Can you work these out from the model? Positions are in its coordinate system, mm. Face numbers are marked on the shaded views. A direction names the side the tool comes from. Give positions to 0.01 mm unless a question says otherwise; leave off trailing zeros. Order: outer loops, then holes, each group sorted by start corner. A loop starts at its lowest first (then second) coordinate and runs counter-clockwise, first axis right, second up.
Item 1: I want a section at B-B, the plane z = 13.25. Write out the boundary of the cut face in (x, y).
Item 2: I want a section at A-A, the plane x = 19. Write out the boundary of the cut face in (y, z).
Item 3: I'm going to push flat-ended pins straight in: pin 1 Ø1 at (x, y) = (-26.5, -22.5) entering from +Z; pin 2 Ø4 at (x, z) = (-13.5, 4) entering from -Y; pin 3 Ø4 at (y, z) = (-19.5, 7.5) entering from -X; pin 4 Ø1.1 at (x, y) = (43.5, 20.5) entering from -Z. Where does each tip first touch, or does it pass through?
Item 4: If I drill on line 1 along Y through (x, z) = (19, 0.7); line 2 along Y through (x, z) = (31, 10.75); line 3 along Z through (x, y) = (-11.5, -1), over which ranges is the centre line in solid material (lowest first)?
Item 5: If we mould it in two halves opening along Y, with no side actions, what happens to the marked faces 1, 2 and 3? For each: +Y half, -Y half, draft (parallel to the pull), parting line (faces both ways), or undercut.
Item 6: I want a section at D-D, the plane x = 38. Write out the boundary of the cut face in (y, z).
Item 7: I want a section at C-C, the plane y = -4. Write out the boundary of the cut face in (x, z), then the cut area to 3 significant figures.
Item 8: Which directions (+Z, -Z, +X, -X, +Y, -Y) give clear straight access to the entire face, cutting with the end or side of a thin tool? Please do the marked faces 4, 5, 6 and 7.
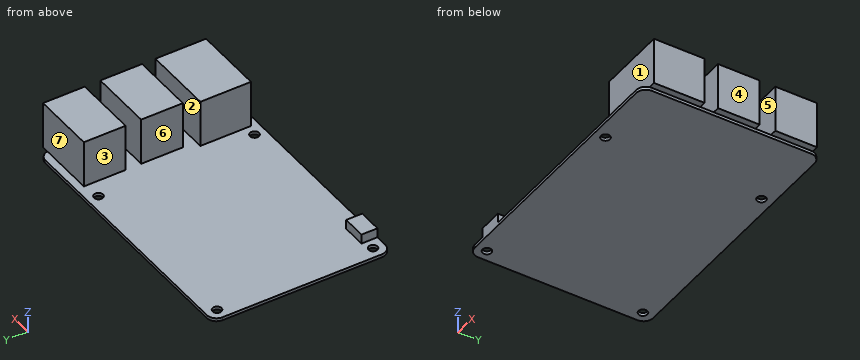
```python
from build123d import *

# Parameters (mm, degrees)
F0_W     = 85
F0_H     = 56
F1_DEPTH = 1
F2_R     = 3
F3_W     = 22
F3_H     = 15.9
F3_W_2   = 20
F3_H_2   = 13.1
F4_DEPTH = 14.8
F6_D     = 2.8
F6_DEPTH = 5
F7_W     = 7.5
F7_H     = 5
F8_DEPTH = 3


with BuildPart() as f1:
    # F0 (on Top) → F1 (new body)
    with BuildSketch(Plane.XY):
        Rectangle(F0_W, F0_H)
    extrude(amount=F1_DEPTH)

    # F2
    f2_edges = [f1.edges().sort_by_distance(p)[0] for p in [
        (42.5, -28, 0.5),
        (42.5, 28, 0.5),
        (-42.5, 28, 0.5),
        (-42.5, -28, 0.5),
    ]]
    fillet(f2_edges, radius=F2_R)

    # F3 (on face) → F4 (join)
    with BuildSketch(Plane.XY.offset(1)):
        with Locations((33.6, -17.75)):
            Rectangle(F3_W, F3_H)
        with Locations((34.6, 0.95)):
            Rectangle(F3_W_2, F3_H_2)
        with Locations((34.6, 18.95)):
            Rectangle(F3_W_2, F3_H_2)
    extrude(amount=F4_DEPTH)

    # F6
    with Locations(Plane.XY.offset(1)):
        with Locations((-39, 24.5), (19, 24.5), (19, -24.5), (-39, -24.5)):
            Hole(F6_D / 2, depth=F6_DEPTH)

    # F7 (on face) → F8 (join)
    with BuildSketch(Plane.XY.offset(1)):
        with Locations((-31.95, -25.5)):
            Rectangle(F7_W, F7_H)
    extrude(amount=F8_DEPTH)


solid = f1.part
```
Results list:
1. outline: (22.6, -25.7) - (44.6, -25.7) - (44.6, -9.8) - (22.6, -9.8) - close; (24.6, -5.6) - (44.6, -5.6) - (44.6, 7.5) - (24.6, 7.5) - close; (24.6, 12.4) - (44.6, 12.4) - (44.6, 25.5) - (24.6, 25.5) - close
2. outline: (-28, 0) - (-25.9, 0) - (-25.9, 1) - (-28, 1) - close; (-23.1, 0) - (23.1, 0) - (23.1, 1) - (-23.1, 1) - close; (25.9, 0) - (28, 0) - (28, 1) - (25.9, 1) - close
3. pin 1: stops at z = 1
3. pin 2: passes through
3. pin 3: stops at x = 22.6
3. pin 4: stops at z = 1
4. line 1: y = -28 to -25.9, -23.1 to 23.1, 25.9 to 28
4. line 2: y = -25.7 to -9.8, -5.6 to 7.5, 12.4 to 25.5
4. line 3: z = 0 to 1
5. face 1: -Y half
5. face 2: undercut
5. face 3: draft
6. outline: (-28, 0) - (28, 0) - (28, 1) - (25.5, 1) - (25.5, 15.8) - (12.4, 15.8) - (12.4, 1) - (7.5, 1) - (7.5, 15.8) - (-5.6, 15.8) - (-5.6, 1) - (-9.8, 1) - (-9.8, 15.8) - (-25.7, 15.8) - (-25.7, 1) - (-28, 1) - close
7. outline: (-42.5, 0) - (42.5, 0) - (42.5, 1) - (44.6, 1) - (44.6, 15.8) - (24.6, 15.8) - (24.6, 1) - (-42.5, 1) - close
7. area: 381 mm2
8. face 4: +Z, -Z, +X, +Y, -Y
8. face 5: +Z, +X, -X
8. face 6: +Z, -X, +Y
8. face 7: +Z, +X, -X, +Y
